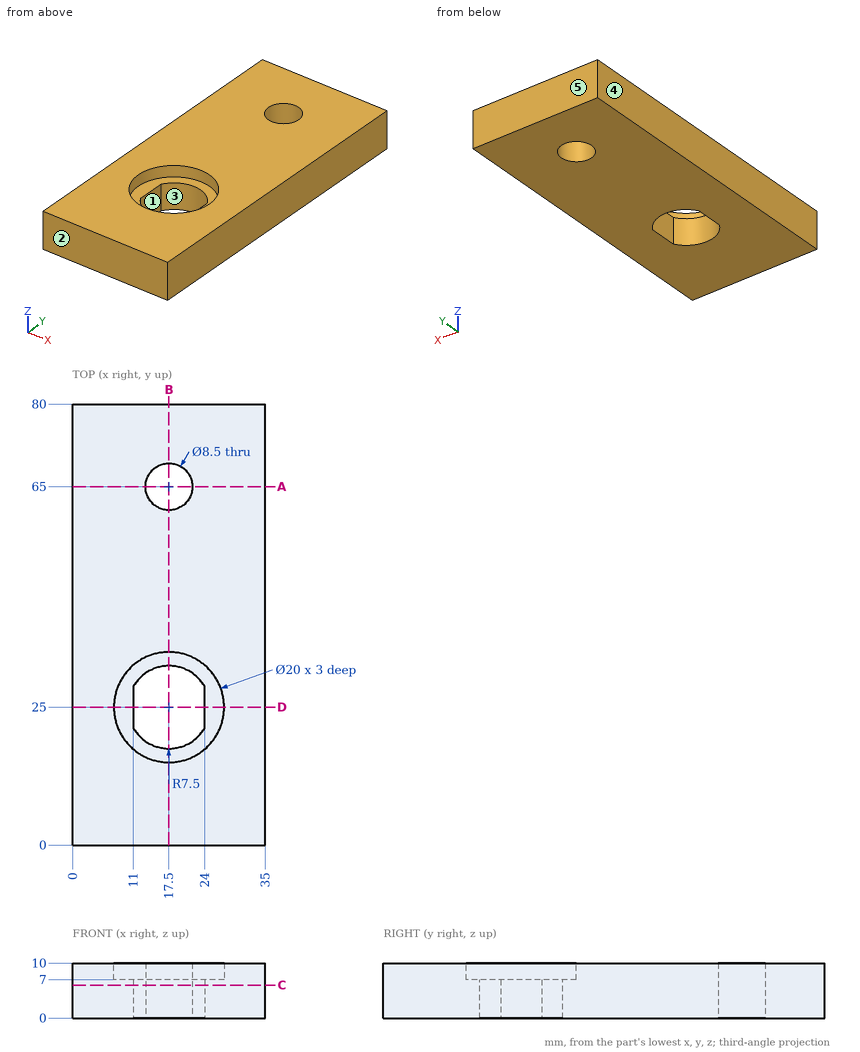
Geometry check sheet. Reference: drawing and pictorial views, mm from the part's lowest x, y, z. A direction names the side the tool comes from. Round coordinates to 2 decimals unless told otherwise and drop trailing zeros. Write each loop counter-clockwise with the first axis right and the second up, starting at its lowest first coordinate (ties: lowest second). Pieces come first, ordered by that corner, then holes.
Item 1: Mould release check, pull along Y, two halves, no side actions. Record for the marked faces 3, 4 and 5: +Y half, -Y half, draft (parallel to the pull), parting line (faces both ways), or undercut.
Determined:
face 3: undercut
face 4: draft
face 5: +Y half
Item 2: Section check B-B (x = 17.5). Record the boundary of the cut face in (y, z), plus the area to 3 significant figures.
Determined:
outline: (0, 0) - (17.5, 0) - (17.5, 7) - (15, 7) - (15, 10) - (0, 10) - close; (32.5, 0) - (60.75, 0) - (60.75, 10) - (35, 10) - (35, 7) - (32.5, 7) - close; (69.25, 0) - (80, 0) - (80, 10) - (69.25, 10) - close
area: 550 mm2
Item 3: Section check A-A (y = 65). Record the boundary of the cut face in (x, z), plus the area to 3 significant figures.
Determined:
outline: (0, 0) - (13.25, 0) - (13.25, 10) - (0, 10) - close; (21.75, 0) - (35, 0) - (35, 10) - (21.75, 10) - close
area: 265 mm2
Item 4: Section check C-C (z = 6). Record the boundary of the cut face in (x, y), plus the area to 3 significant figures.
Determined:
outline: (0, 0) - (35, 0) - (35, 80) - (0, 80) - close; hole (11, 21.26) arc R7.5 ccw to (24, 21.26) - (24, 28.74) arc R7.5 ccw to (11, 28.74) - close; hole circle Ø8.5 at (17.5, 65)
area: 2,580 mm2
Item 5: Access from +Z, -Z, +X, -X, +Y, -Y to the whole of each face (thin tool, end or side, straight path). Record for the marked faces 1 and 2.
Determined:
face 1: +Z, -Z
face 2: +Z, -Z, +X, -X, -Y
Item 6: Material ranges on line 1 along Y through (x, z) = (17.5, 8.85); line 2 along X through (y, z) = (23.5, 3); line 3 along Y through (x, z) = (19, 3), recorded low to high.
Determined:
line 1: y = 0 to 15, 35 to 60.75, 69.25 to 80
line 2: x = 0 to 11, 24 to 35
line 3: y = 0 to 17.65, 32.35 to 61.02, 68.98 to 80
Item 7: Section check D-D (y = 25). Record the boundary of the cut face in (x, z), plus the area to 3 significant figures.
Determined:
outline: (0, 0) - (11, 0) - (11, 7) - (7.5, 7) - (7.5, 10) - (0, 10) - close; (24, 0) - (35, 0) - (35, 10) - (27.5, 10) - (27.5, 7) - (24, 7) - close
area: 199 mm2
Item 8: Go/stop test with a flat-tipped pin: pin 1 Ø5 at (x, y) = (17.5, 65) entering from +Z. Record where the tip stops, or that it passes through.
Determined:
pin 1: passes through
